```python
from build123d import *

# Parameters (mm, degrees)
SALIENTE_EXTRUIR1_DEPTH = 38.1
SALIENTE_EXTRUIR2_DEPTH = 1


with BuildPart() as part:
    # Croquis1 → Saliente-Extruir1 (new body)
    with BuildSketch(Plane.XY):
        with BuildLine():
            Line((-6.828427125, 6.828427125), (-63.639610307, 63.639610307))
            Line((-63.639610307, 63.639610307), (-62.225396744, 65.053823869))
            Line((-62.225396744, 65.053823869), (-5.414213562, 8.242640687))
            ThreePointArc((-5.414213562, 8.242640687), (-4.113577054, 1.703899406), (-9.656854249, -2))
            Line((-9.656854249, -2), (-90, -2))
            Line((-90, -2), (-90, 0))
            Line((-90, 0), (-9.656854249, 0))
            ThreePointArc((-9.656854249, 0), (-5.961336119, 2.469266271), (-6.828427125, 6.828427125))
        make_face()
    extrude(amount=SALIENTE_EXTRUIR1_DEPTH)

    # Croquis3 → Saliente-Extruir2 (add, symmetric)
    with BuildSketch(Plane.XY.offset(19.05)):
        Polygon((-40.597622613, 0), (-20.298811306, 20.298811306), (-6.828427125, 6.828427125), (-13.656854249, 0), align=None)
    extrude(amount=SALIENTE_EXTRUIR2_DEPTH, both=True)


solid = part.part
```
Verification items for the finished model (mm, model axes). A direction names the side the tool comes from. Give positions to 0.01 mm unless a question says otherwise; leave off trailing zeros. Order: outer loops, then holes, each group sorted by start corner. A loop starts at its lowest first (then second) coordinate and runs counter-clockwise, first axis right, second up. Notation, with made-up numbers: (-12, 83.25) -> (19, 83.25) arc R11 cw to (19, 99.25) -> close; hole circle Ø3 at (-13, -31). An arc over 180 degrees is marked (long way). Use a Markdown table: item, result.
1) Depth check by flat-ended pin: pin 1 Ø10 at (x, y) = (-20, 7.5) entering from -Z; pin 2 Ø6 at (y, z) = (40.5, 9) entering from -X; pin 3 Ø8 at (y, z) = (22.5, 13) entering from +X; pin 4 Ø22.5 at (x, y) = (-17, 15) entering from +Z. Enter the tip coordinate at first touch or a pass-through.
Results:
| item | result |
|---|---|
| pin 1 | z = 18.05 |
| pin 2 | x = -43.5 |
| pin 3 | x = -15.67 |
| pin 4 | z = 38.1 |
2) Section check C-C, the plane z = 6.5. Record the boundary of the cut face in (x, y), then the cut area to 3 significant figures.
Results:
| item | result |
|---|---|
| outline | (-90, -2) -> (-9.66, -2) arc R6 ccw to (-5.41, 8.24) -> (-62.23, 65.05) -> (-63.64, 63.64) -> (-6.83, 6.83) arc R4 cw to (-9.66, 0) -> (-90, 0) -> close |
| area | 345 mm² |
3) Section check B-B, the plane x = -26. Record the boundary of the cut face in (y, z).
Results:
| item | result |
|---|---|
| outline | (-2, 0) -> (0, 0) -> (0, 18.05) -> (14.6, 18.05) -> (14.6, 20.05) -> (0, 20.05) -> (0, 38.1) -> (-2, 38.1) -> close; (26, 0) -> (28.83, 0) -> (28.83, 38.1) -> (26, 38.1) -> close |
4) Tool access check on faces 4 (the flat face through (-30.6, 10, 19.1)), 5 (the flat face through (-23, 8, 20.05)), 6 (the flat face through (-23, 8, 18.05)). Record the directions out of +Z, -Z, +X, -X, +Y, -Y that give a thin tool (end or side, any length) a straight path to the whole face; none if there is none.
Results:
| item | result |
|---|---|
| face 4 | +Z, -Z, -X |
| face 5 | +Z, -X |
| face 6 | -Z, -X |
5) Material ranges on probe 1 along Z at (x, y) = (-28.5, 12); probe 2 along Y at (x, z) = (-38, 6); probe 3 along Y at (x, z) = (-25.5, 16), recorded low to high.
Results:
| item | result |
|---|---|
| probe 1 | 18.05 to 20.05 |
| probe 2 | -2 to 0, 38 to 40.83 |
| probe 3 | -2 to 0, 25.5 to 28.33 |
6) Section check A-A, the plane z = 19. Record the boundary of the cut face in (x, y), then the cut area to 3 significant figures.
Results:
| item | result |
|---|---|
| outline | (-90, -2) -> (-9.66, -2) arc R6 ccw to (-5.41, 8.24) -> (-62.23, 65.05) -> (-63.64, 63.64) -> (-20.3, 20.3) -> (-40.6, 0) -> (-90, 0) -> close; hole (-13.66, 0) -> (-9.66, 0) arc R4 ccw to (-6.83, 6.83) -> close |
| area | 710 mm² |
7) Mould release check, pull along Y, two halves, no side actions. Record for faces 1 (the flat face through (-34.22, 37.05, 18.78)), 2 (the flat face through (-10.195, 3.462, 19.064)), 3 (the flat face through (-90, -1, 19)): pulls with the +Y half, pulls with the -Y half, needs draft (parallel to the pull), parting line crosses it, or undercut.
Results:
| item | result |
|---|---|
| face 1 | pulls with the +Y half |
| face 2 | undercut |
| face 3 | needs draft |
8) Section check D-D, the plane y = 10. Record the boundary of the cut face in (x, z), then the cut area to 3 significant figures.
Results:
| item | result |
|---|---|
| outline | (-30.6, 18.05) -> (-10, 18.05) -> (-10, 0) -> (-7.17, 0) -> (-7.17, 38.1) -> (-10, 38.1) -> (-10, 20.05) -> (-30.6, 20.05) -> close |
| area | 149 mm² |
